```python
from build123d import *

# Parameters (mm, degrees)
F0_W     = 254
F0_H     = 254
F1_DEPTH = 15.875
F2_R     = 101.6


with BuildPart() as f1:
    # F0 (on Front) → F1 (new body)
    with BuildSketch(Plane.XZ):
        Polygon((304.8, -508), (304.8, 508), (127, 508), (-127, 508), (-304.8, 508), (-304.8, -508), align=None)
        with Locations((0, 635)):
            Rectangle(F0_W, F0_H)
    extrude(amount=F1_DEPTH)

    # F2
    f2_edges = [f1.edges().sort_by_distance(p)[0] for p in [
        (127, -7.9375, 762),
        (304.8, -7.9375, 508),
        (-304.8, -7.9375, 508),
        (-127, -7.9375, 762),
    ]]
    fillet(f2_edges, radius=F2_R)


solid = f1.part
```
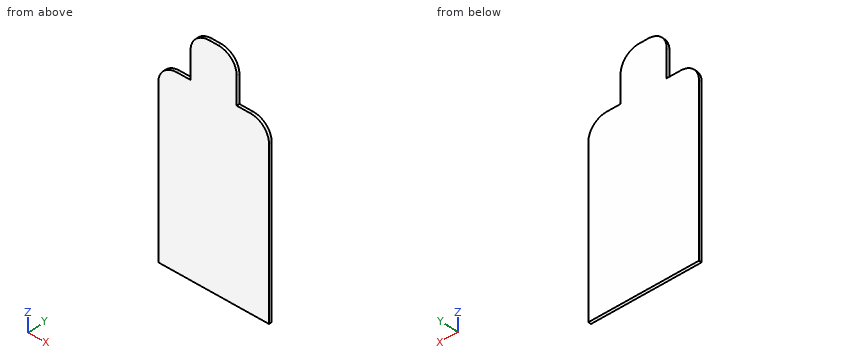
Read the model definition and answer for the solid it produces. Units are mm, in the model's axes. Give positions to 0.01 mm unless a question says otherwise; leave off trailing zeros. Order: outer loops, then holes, each group sorted by start corner. A loop starts at its lowest first (then second) coordinate and runs counter-clockwise, first axis right, second up. Notation, with made-up numbers: (-8, -4) -> (31, -4) arc R26 cw to (31, 16) -> close; hole circle Ø7 at (79, 14). An arc over 180 degrees is marked (long way). One line per item, written item: value. Start each with the question number.
(1) The part is cut by section C-C (z = 609.5). Determine the outline of the cut face in (x, y) (3 decimals).
(2) Straight lines are drawn through the part: L1, parallel to Z at x = 192, y = -11.5; L2, parallel to Z at x = 252, y = -10.5; L3, parallel to X at y = -3, z = 691. For each, find the intervals that lie inside material, in ascending order.
(3) Flat-ended cylindrical pins translate along their axes: P1, Ø3, axis at y = -2.5, z = 477, coming from the +X side; P2, Ø8, axis at x = -175, y = -7, coming from the +Z side; P3, Ø8, axis at x = -82.5, z = 621.5, coming from the +Y side; P4, Ø8, axis at x = 60.5, y = -8.5, coming from the +Z side. Find the tip coordinate at first contact, or state that the pin passes through.
(4) The part is cut by section A-A (y = -11). Determine the outline of the cut face in (x, z), and give its area (3 significant figures).
(5) The part is cut by section B-B (x = 173). Determine the outline of the cut face in (y, z) (3 decimals).
Taken from the geometry:
1. outline: (-127, -15.875) -> (127, -15.875) -> (127, 0) -> (-127, 0) -> close
2. L1: -508 to 508
2. L2: -508 to 495.51
2. L3: -122.28 to 122.28
3. P1: x = 277.68
3. P2: z = 508
3. P3: y = 0
3. P4: z = 757.12
4. outline: (-304.8, -508) -> (304.8, -508) -> (304.8, 406.4) arc R101.6 ccw to (203.2, 508) -> (127, 508) -> (127, 660.4) arc R101.6 ccw to (25.4, 762) -> (-25.4, 762) arc R101.6 ccw to (-127, 660.4) -> (-127, 508) -> (-203.2, 508) arc R101.6 ccw to (-304.8, 406.4) -> close
4. area: 675,000 mm^2
5. outline: (-15.875, -508) -> (0, -508) -> (0, 508) -> (-15.875, 508) -> close
